```python
from build123d import *

# Parameters (mm, degrees)
BOSS_EXTRUDE1_DEPTH = 3
FILLET1_R           = 20
FILLET2_R           = 10
FILLET3_R           = 6
BOSS_EXTRUDE2_START = 5
BOSS_EXTRUDE2_DEPTH = 5
BOSS_EXTRUDE3_DEPTH = 5


with BuildPart() as part:
    # Sketch1 → Boss-Extrude1 (new body)
    with BuildSketch(Plane.XY):
        with BuildLine():
            Line((58.995636199, -70), (85.000010905, 5.7991e-05))
            add(Edge.make_bspline(
                [(85.000010905, 5.7991e-05), (56.750474686, 7.0174992), (28.420775895, 13.71150164), (7.678e-06, 19.999882532)],
                knots=[0, 0, 0, 0, 1, 1, 1, 1], degree=3))
            add(Edge.make_bspline(
                [(7.678e-06, 19.999882532), (-28.420729921, 13.711538103), (-56.750527687, 7.017544413), (-85.000042152, 0.000142104)],
                knots=[0, 0, 0, 0, 1, 1, 1, 1], degree=3))
            Line((-85.000042152, 0.000142104), (-58.995636199, -70))
            Line((-58.995636199, -70), (0, -80))
            Line((0, -80), (58.995636199, -70))
        make_face()
        with BuildLine():
            Line((51.632125707, -61.105504126), (71.72329576, -7.02294745))
            add(Edge.make_bspline(
                [(71.72329576, -7.02294745), (65.760246295, -5.560581522), (53.826176048, -2.665485282), (35.906371118, 1.582198174), (17.96537234, 5.730748209), (5.991311045, 8.427016674), (2.578e-06, 9.757206823)],
                knots=[0.12850852, 0.12850852, 0.12850852, 0.12850852, 0.340025725, 0.551542931, 0.763060137, 0.974577343, 0.974577343, 0.974577343, 0.974577343], degree=3))
            add(Edge.make_bspline(
                [(2.578e-06, 9.757206823), (-5.991303797, 8.427023399), (-17.965355756, 5.730769647), (-35.906372035, 1.582235194), (-53.826198007, -2.665432907), (-65.760270504, -5.560515659), (-71.723322613, -7.022875166)],
                knots=[0.025422687, 0.025422687, 0.025422687, 0.025422687, 0.236939832, 0.448456977, 0.659974121, 0.871491266, 0.871491266, 0.871491266, 0.871491266], degree=3))
            Line((-71.723322613, -7.022875166), (-51.632125707, -61.105504126))
            Line((-51.632125707, -61.105504126), (0, -69.857359184))
            Line((0, -69.857359184), (51.632125707, -61.105504126))
        make_face(mode=Mode.SUBTRACT)
    extrude(amount=BOSS_EXTRUDE1_DEPTH)

    # Fillet1
    fillet1_edges = [part.edges().sort_by_distance(p)[0] for p in [
        (0, -69.857359184, 1.5),
        (2.578e-06, 9.757206823, 1.5),
    ]]
    fillet(fillet1_edges, radius=FILLET1_R)

    # Fillet2
    fillet2_edges = [part.edges().sort_by_distance(p)[0] for p in [
        (51.632125707, -61.105504126, 1.5),
        (-51.632125707, -61.105504126, 1.5),
    ]]
    fillet(fillet2_edges, radius=FILLET2_R)

    # Fillet3
    fillet3_edges = [part.edges().sort_by_distance(p)[0] for p in [
        (71.72329576, -7.02294745, 1.5),
        (-71.723322613, -7.022875166, 1.5),
    ]]
    fillet(fillet3_edges, radius=FILLET3_R)

    # Sketch2 → Boss-Extrude2 (add)
    with BuildSketch(Plane.XY.offset(3).offset(BOSS_EXTRUDE2_START)):
        with BuildLine():
            Line((-81.681959277, -1.75265922), (-57.154758576, -67.776376032))
            Line((-57.154758576, -67.776376032), (0, -77.464339796))
            Line((0, -77.464339796), (57.154758576, -67.776376032))
            Line((57.154758576, -67.776376032), (81.681929126, -1.752740382))
            add(Edge.make_bspline(
                [(81.681929126, -1.752740382), (54.532239341, 4.970251393), (27.308171531, 11.391977282), (6.404e-06, 17.439367697)],
                knots=[0, 0, 0, 0, 1, 1, 1, 1], degree=3))
            add(Edge.make_bspline(
                [(6.404e-06, 17.439367697), (-27.308135136, 11.392011032), (-54.532288876, 4.970295529), (-81.681959277, -1.75265922)],
                knots=[0, 0, 0, 0, 1, 1, 1, 1], degree=3))
        make_face()
        with BuildLine():
            Line((-69.376008475, -13.341509152), (-53.642677645, -55.693385824))
            ThreePointArc((-53.642677645, -55.693385824), (-50.645602116, -59.913867336), (-45.939817671, -62.070373463))
            Line((-45.939817671, -62.070373463), (-3.342404912, -69.290807973))
            ThreePointArc((-3.342404912, -69.290807973), (0, -69.572077553), (3.342404912, -69.290807973))
            Line((3.342404912, -69.290807973), (45.939817671, -62.070373463))
            ThreePointArc((45.939817671, -62.070373463), (50.645602116, -59.913867336), (53.642677645, -55.693385824))
            Line((53.642677645, -55.693385824), (69.375984259, -13.341574337))
            ThreePointArc((69.375984259, -13.341574337), (69.05053211, -8.437764256), (65.169862303, -5.422192294))
            add(Edge.make_bspline(
                [(65.169862303, -5.422192294), (61.388993913, -4.502380085), (51.638475989, -2.146916169), (35.906371118, 1.582198174), (19.417348722, 5.39500343), (8.898318707, 7.771361324), (4.363182833, 8.785163741)],
                knots=[0.205976361, 0.205976361, 0.205976361, 0.205976361, 0.340025725, 0.551542931, 0.763060137, 0.923222679, 0.923222679, 0.923222679, 0.923222679], degree=3))
            ThreePointArc((4.363182833, 8.785163741), (2.348e-06, 9.266901295), (-4.363178618, 8.785168098))
            add(Edge.make_bspline(
                [(-4.363178618, 8.785168098), (-8.898311373, 7.771371135), (-19.41733449, 5.395025913), (-35.906372035, 1.582235194), (-51.638493171, -2.146865145), (-61.389012491, -4.502317987), (-65.169880027, -5.422125529)],
                knots=[0.076777369, 0.076777369, 0.076777369, 0.076777369, 0.236939832, 0.448456977, 0.659974121, 0.794023369, 0.794023369, 0.794023369, 0.794023369], degree=3))
            ThreePointArc((-65.169880027, -5.422125529), (-69.050554759, -8.437696121), (-69.376008475, -13.341509152))
        make_face(mode=Mode.SUBTRACT)
    extrude(amount=-BOSS_EXTRUDE2_DEPTH)

    # Sketch3 → Boss-Extrude3 (add)
    with BuildSketch(Plane(origin=(0, 0, 0), x_dir=(-1, 0, 0), z_dir=(0, 0, -1))):
        with BuildLine():
            Line((57.522934276, -68.221100795), (82.345641792, -1.401949233))
            add(Edge.make_bspline(
                [(82.345641792, -1.401949233), (54.976968444, 5.379009049), (27.531586141, 11.851868369), (0.000183244, 17.939432259)],
                knots=[-0.01124673, -0.01124673, -0.01124673, -0.01124673, 1.075105268, 1.075105268, 1.075105268, 1.075105268], degree=3))
            add(Edge.make_bspline(
                [(0.000183244, 17.939432259), (-27.531342023, 11.851872874), (-54.976750263, 5.379036047), (-82.345641148, -1.401950967)],
                knots=[-0.075105482, -0.075105482, -0.075105482, -0.075105482, 1.011252332, 1.011252332, 1.011252332, 1.011252332], degree=3))
            Line((-82.345641148, -1.401950967), (-57.522934276, -68.221100795))
            Line((-57.522934276, -68.221100795), (0, -77.971471837))
            Line((0, -77.971471837), (57.522934276, -68.221100795))
        make_face()
        with BuildLine():
            Line((-53.642677645, -55.693385824), (-69.375984259, -13.341574337))
            ThreePointArc((-69.375984259, -13.341574337), (-69.05053211, -8.437764256), (-65.169862303, -5.422192294))
            add(Edge.make_bspline(
                [(-65.169862303, -5.422192294), (-61.388993913, -4.502380085), (-51.638475989, -2.146916169), (-35.906371118, 1.582198174), (-19.417348722, 5.39500343), (-8.898318707, 7.771361324), (-4.363182833, 8.785163741)],
                knots=[0.205976361, 0.205976361, 0.205976361, 0.205976361, 0.340025725, 0.551542931, 0.763060137, 0.923222679, 0.923222679, 0.923222679, 0.923222679], degree=3))
            ThreePointArc((-4.363182833, 8.785163741), (-2.348e-06, 9.266901295), (4.363178618, 8.785168098))
            add(Edge.make_bspline(
                [(4.363178618, 8.785168098), (8.898311373, 7.771371135), (19.41733449, 5.395025913), (35.906372035, 1.582235194), (51.638493171, -2.146865145), (61.389012491, -4.502317987), (65.169880027, -5.422125529)],
                knots=[0.076777369, 0.076777369, 0.076777369, 0.076777369, 0.236939832, 0.448456977, 0.659974121, 0.794023369, 0.794023369, 0.794023369, 0.794023369], degree=3))
            ThreePointArc((65.169880027, -5.422125529), (69.050554759, -8.437696121), (69.376008475, -13.341509152))
            Line((69.376008475, -13.341509152), (53.642677645, -55.693385824))
            ThreePointArc((53.642677645, -55.693385824), (50.645602116, -59.913867336), (45.939817671, -62.070373463))
            Line((45.939817671, -62.070373463), (3.342404912, -69.290807973))
            ThreePointArc((3.342404912, -69.290807973), (0, -69.572077553), (-3.342404912, -69.290807973))
            Line((-3.342404912, -69.290807973), (-45.939817671, -62.070373463))
            ThreePointArc((-45.939817671, -62.070373463), (-50.645602116, -59.913867336), (-53.642677645, -55.693385824))
        make_face(mode=Mode.SUBTRACT)
    extrude(amount=BOSS_EXTRUDE3_DEPTH)


solid = part.part
```
Check sheet for the modelled part. Datum: model origin and axes. Units: mm. A direction names the side the tool comes from. Coordinates: 2 decimals unless noted, no trailing zeros. Order: outer loops, then holes, each group sorted by start corner. A loop starts at its lowest first (then second) coordinate and runs counter-clockwise, first axis right, second up. Notation, with made-up numbers: M 21.25,-27 L 78.25,-27 A9 ccw 78.25,-22 Z; hole C 24,69 d7. An arc over 180 degrees is marked long. Write each question's results on one line, items separated by ' | '. Start each with the question number.
1. Cross-section at B-B on y = -44. Record the cut outline in (x, z).
2. Cross-section at A-A on y = -64. Record the cut outline in (x, z).
3. Mould release check, pull along Y, two halves, no side actions. Record for faces 1 (the face through (-6, 9, 8)), 2 (the face through (0.062, 9.267, -2.465)), 3 (the face through (70.11, -34.34, -2.46)): +Y half, -Y half, draft (parallel to the pull), parting line (faces both ways), or undercut.
4. Go/stop test with flat-tipped pins: P1, Ø1.5, axis at x = -22, z = -1.5, coming from the +Y side; P2, Ø4, axis at y = -27, z = -3.5, coming from the -X side; P3, Ø3, axis at y = -15.5, z = 2, coming from the +X side. Record where each tip stops, or that it passes through.
5. Material ranges on probe 1 along X at (y, z) = (-30.5, 1.5); probe 2 along X at (y, z) = (-35, 4.25); probe 3 along Y at (x, z) = (-10.5, 3.5), recorded low to high.
6. Access from +Z, -Z, +X, -X, +Y, -Y to the whole of each face (thin tool, end or side, straight path). Record for faces 4 (the face through (0.062, 9.267, 5.535)), 5 (the face through (-69.76, -35.28, -2.46)), 6 (the face through (-28.977, -72.553, 5.535)).
Checks:
1) outline: M -68.65,0 L -66.52,0 L -66.52,-5 L -57.99,-5 L -57.99,8 L -65.99,8 L -65.99,3 L -68.65,3 Z; M 57.99,-5 L 66.52,-5 L 66.52,0 L 68.65,0 L 68.65,3 L 65.99,3 L 65.99,8 L 57.99,8 Z
2) outline: M -61.22,0 L -59.09,0 L -59.09,-5 L -34.56,-5 L -34.56,8 L -58.56,8 L -58.56,3 L -61.22,3 Z; M 34.56,-5 L 59.09,-5 L 59.09,0 L 61.22,0 L 61.22,3 L 58.56,3 L 58.56,8 L 34.56,8 Z
3) face 1: draft | face 2: undercut | face 3: -Y half
4) P1: stops at y = 13.16 | P2: stops at x = -73.58 | P3: stops at x = 79.8
5) probe 1: x = -73.67 to -63, 63 to 73.67 | probe 2: x = -69.33 to -61.33, 61.33 to 69.33 | probe 3: y = -75.68 to -68.08, 7.41 to 15.09
6) face 4: +Z, -Z | face 5: -Z, -X, -Y | face 6: +Z, -X, -Y
